Build history of the part. All positions in model axes, mm. A direction names the side the tool comes from. Coordinates: 2 decimals unless noted, no trailing zeros. Order: outer loops, then holes, each group sorted by start corner. A loop starts at its lowest first (then second) coordinate and runs counter-clockwise, first axis right, second up. Notation, with made-up numbers: (6, 72) - (58, 72) arc R29 ccw to (58, 99) - close; hole circle Ø11 at (1.5, 2.5). An arc over 180 degrees is marked (long way). One line per item, written item: value.
from build123d import *

# Parameters (mm, degrees)
SKETCH_R     = 1.6
SKETCH_R_2   = 2.1
SKETCH_R_3   = 3.75
SKETCH_W     = 6.5
SKETCH_H     = 4
PAD_DEPTH    = 10
SKETCH001_R  = 4
POCKET_DEPTH = 4
FILLET_R     = 6
FILLET001_R  = 4.99


with BuildPart() as part:
    # Sketch → Pad (new body)
    with BuildSketch(Plane.XY):
        Polygon((-38.5, 40), (-38.5, -40), (-38.5, -45), (-13.5, -45), (-13.5, -40), (38.5, -40), (38.5, 40), (-13.5, 40), (-13.5, 45), (-38.5, 45), align=None)
        with Locations((-15, 0)):
            Circle(SKETCH_R, mode=Mode.SUBTRACT)
        with Locations((15, -30)):
            Circle(SKETCH_R, mode=Mode.SUBTRACT)
        with Locations((0, 20)):
            Circle(SKETCH_R_2, mode=Mode.SUBTRACT)
        with Locations((0, -20)):
            Circle(SKETCH_R_2, mode=Mode.SUBTRACT)
        with Locations((15, 30)):
            Circle(SKETCH_R, mode=Mode.SUBTRACT)
        with Locations((-17.5, 17.5)):
            Circle(SKETCH_R_3, mode=Mode.SUBTRACT)
        with Locations((-17.5, -17.5)):
            Circle(SKETCH_R_3, mode=Mode.SUBTRACT)
        with Locations((17.5, -17.5)):
            Circle(SKETCH_R_3, mode=Mode.SUBTRACT)
        with Locations((17.5, 17.5)):
            Circle(SKETCH_R_3, mode=Mode.SUBTRACT)
        with Locations((0, 4)):
            Rectangle(SKETCH_W, SKETCH_H, mode=Mode.SUBTRACT)
        with Locations((0, -4)):
            Rectangle(SKETCH_W, SKETCH_H, mode=Mode.SUBTRACT)
        with Locations((0, 12)):
            Rectangle(SKETCH_W, SKETCH_H, mode=Mode.SUBTRACT)
        with Locations((0, -12)):
            Rectangle(SKETCH_W, SKETCH_H, mode=Mode.SUBTRACT)
    extrude(amount=PAD_DEPTH)

    # Sketch001 (on Face34 of Pad) → Pocket (cut)
    with BuildSketch(Plane.XY.offset(10)):
        with Locations((-15, 0)):
            Circle(SKETCH001_R)
        with Locations((15, -30)):
            Circle(SKETCH001_R)
        with Locations((15, 30)):
            Circle(SKETCH001_R)
        with Locations((0, 20)):
            Circle(SKETCH001_R)
        with Locations((0, -20)):
            Circle(SKETCH001_R)
    extrude(amount=-POCKET_DEPTH, mode=Mode.SUBTRACT)

    # Fillet
    fillet_edges = [part.edges().sort_by_distance(p)[0] for p in [
        (-38.5, -45, 5),
        (38.5, -40, 5),
        (-38.5, 45, 5),
        (38.5, 40, 5),
    ]]
    fillet(fillet_edges, radius=FILLET_R)

    # Fillet001
    fillet001_edges = [part.edges().sort_by_distance(p)[0] for p in [
        (-13.5, 45, 5),
        (-13.5, -45, 5),
    ]]
    fillet(fillet001_edges, radius=FILLET001_R)


solid = part.part
1. Band-saw the part on D-D, the plane z = 7.75. Count the separate pieces of the cut face and the enclosed holes in it, and give its area (3 significant figures).
Values found:
separate pieces: 1
enclosed holes: 13
area: 5,840 mm2
2. Band-saw the part on C-C, the plane y = 20. Give the cut face in (x, z).
Values found:
outline: (-38.5, 0) - (-20.3, 0) - (-20.3, 10) - (-38.5, 10) - close; (-14.7, 0) - (-2.1, 0) - (-2.1, 6) - (-4, 6) - (-4, 10) - (-14.7, 10) - close; (2.1, 0) - (14.7, 0) - (14.7, 10) - (4, 10) - (4, 6) - (2.1, 6) - close; (20.3, 0) - (38.5, 0) - (38.5, 10) - (20.3, 10) - close
3. Band-saw the part on A-A, the plane y = -30. Give the cut face in (x, z).
Values found:
outline: (-38.5, 0) - (13.4, 0) - (13.4, 6) - (11, 6) - (11, 10) - (-38.5, 10) - close; (16.6, 0) - (38.5, 0) - (38.5, 10) - (19, 10) - (19, 6) - (16.6, 6) - close
4. 3-axis set-ups, long thin cutter, end or side, ignore diameter. For faces 1 (the face through (-1, 1, 0)), 2 (the face through (0, -2, 5)), 3 (the face through (-19, 0, 8)): which of +Z, -Z, +X, -X, +Y, -Y reach the whole face in a straight line?
Values found:
face 1: -Z, +X, -X, +Y, -Y
face 2: +Z, -Z
face 3: +Z
5. Band-saw the part on B-B, the plane x = -15. Give the cut face in (y, z), and give its area (3 significant figures).
Values found:
outline: (-43.58, 0) - (-20.3, 0) - (-20.3, 10) - (-43.58, 10) - close; (-14.7, 0) - (-1.6, 0) - (-1.6, 6) - (-4, 6) - (-4, 10) - (-14.7, 10) - close; (1.6, 0) - (14.7, 0) - (14.7, 10) - (4, 10) - (4, 6) - (1.6, 6) - close; (20.3, 0) - (43.58, 0) - (43.58, 10) - (20.3, 10) - close
area: 709 mm2
6. Flat gauge pins, fed straight in: P1, Ø4, axis at x = 18.5, z = 8, coming from the +Y side; P2, Ø3, axis at x = 10.5, z = 4.5, coming from the -Y side; P3, Ø6.5, axis at x = 0, y = 20, coming from the +Z side. Where does each tip first touch, or does it go through?
Values found:
P1: stops at y = 40
P2: stops at y = -40
P3: stops at z = 6
7. Probe line 1 along X through (y, z) = (13, 7.25); line 2 along X through (y, z) = (-20, 2.9); line 3 along X through (y, z) = (0, 2.4). List the from-to ranges inside material, lowest first.
Values found:
line 1: x = -38.5 to -3.25, 3.25 to 38.5
line 2: x = -38.5 to -20.3, -14.7 to -2.1, 2.1 to 14.7, 20.3 to 38.5
line 3: x = -38.5 to -16.6, -13.4 to 38.5
8. Two-plate mould, pull along Y, no slides. Class faces 4 (the face through (-25, 45, 5)), 5 (the face through (17, -30, 6)), 6 (the face through (9, -40, 5)): pulls with the +Y half, pulls with the -Y half, needs draft (parallel to the pull), parting line crosses it, or undercut.
Values found:
face 4: pulls with the +Y half
face 5: undercut
face 6: pulls with the -Y half
